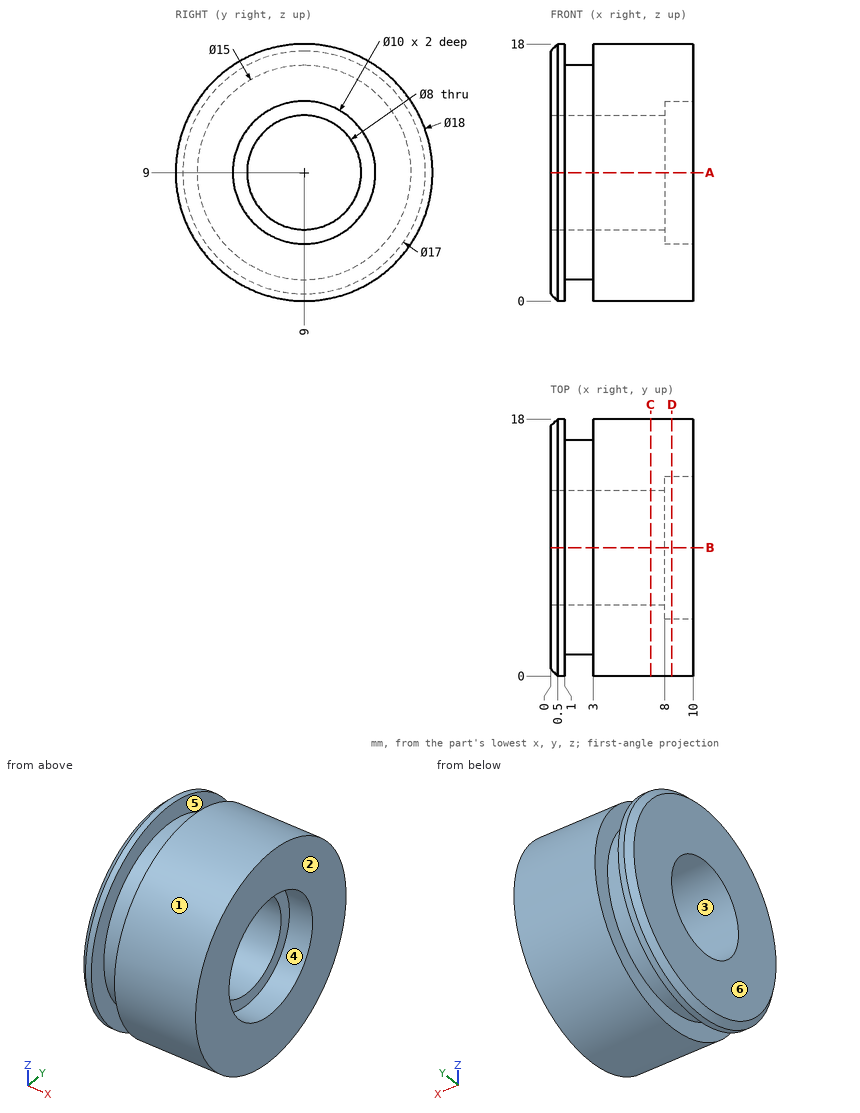
Print and shaded views of the part. All mm, measured from the part's lowest x, y and z. A direction names the side the tool comes from. Round coordinates to 2 decimals unless told otherwise and drop trailing zeros. Write each loop counter-clockwise with the first axis right and the second up, starting at its lowest first coordinate (ties: lowest second). Pieces come first, ordered by that corner, then holes. Notation, with made-up numbers: (71.5, 8) -> (128.5, 8) arc R13 ccw to (128.5, 15) -> close; hole circle Ø5 at (68.5, -35.5). An arc over 180 degrees is marked (long way). Write item = value, one per line.
(1) Probe L1, parallel to X at y = 13.75, z = 16; L2, parallel to Y at x = 9.35, z = 9; L3, parallel to Y at x = 6, z = 9. List the from-to ranges inside material, lowest first.
Answer:
L1 = 0 to 1, 3 to 10
L2 = 0 to 4, 14 to 18
L3 = 0 to 5, 13 to 18
(2) Tool access for the marked faces 4, 5 and 6: list every direction of +Z, -Z, +X, -X, +Y, -Y with a clear straight run to the whole face (end or side of a thin tool).
Answer:
face_4 = +X
face_5 = none
face_6 = +Z, -Z, -X, +Y, -Y
(3) Band-saw the part on A-A (z = 9). Give the cut face in (x, y).
Answer:
outline = (0, 0.5) -> (0.5, 0) -> (1, 0) -> (1, 1.5) -> (3, 1.5) -> (3, 0) -> (10, 0) -> (10, 4) -> (8, 4) -> (8, 5) -> (0, 5) -> close; (0, 13) -> (8, 13) -> (8, 14) -> (10, 14) -> (10, 18) -> (3, 18) -> (3, 16.5) -> (1, 16.5) -> (1, 18) -> (0.5, 18) -> (0, 17.5) -> close
(4) Two-plate mould, pull along Y, no slides. Class the marked faces 1, 2 and 3: pulls with the +Y half, pulls with the -Y half, needs draft (parallel to the pull), parting line crosses it, or undercut.
Answer:
face_1 = parting line crosses it
face_2 = needs draft
face_3 = undercut
(5) Band-saw the part on D-D (x = 8.5). Give the cut face in (y, z), then the cut area to 3 significant figures.
Answer:
outline = circle Ø18 at (9, 9); hole circle Ø10 at (9, 9)
area = 176 mm2
(6) Band-saw the part on C-C (x = 7). Give the cut face in (y, z).
Answer:
outline = circle Ø18 at (9, 9); hole circle Ø8 at (9, 9)
(7) Flat gauge pins, fed straight in: pin 1 (4 mm diameter, centred on x = 1.5, z = 6.5, fed in from +Y); pin 2 (5 mm diameter, centred on y = 7.5, z = 10.5, fed in from +X); pin 3 (1 mm diameter, centred on x = 4, z = 12, fed in from -Y); pin 4 (9 mm diameter, centred on y = 8, z = 5, fed in from +X). Where does each tip first touch, or does it go through?
Answer:
pin_1 = 17.98
pin_2 = 8
pin_3 = 0.35
pin_4 = 10
